from build123d import *

# Parameters (mm, degrees)
F3_D           = 4.4
F3_CSINK_D     = 8.96
F3_CSINK_ANGLE = 90
F4_SIZE        = 1


with BuildPart() as f1:
    # F0 (on Front) → F1 (revolve)
    with BuildSketch(Plane.XZ):
        Polygon((0, 8), (0, 0), (3.5, 0), (3.5, 5), (7.5, 5), (7.5, 8), align=None)
    revolve(axis=Axis((0, 0, 4), (0, 0, 1)))

    # F3 (through all)
    with Locations(Plane.XY.offset(8)):
        with Locations((0, 0)):
            CounterSinkHole(F3_D / 2, F3_CSINK_D / 2, counter_sink_angle=F3_CSINK_ANGLE)

    # F4
    f4_edges = [f1.edges().sort_by_distance(p)[0] for p in [
        (-7.5, 0, 5),
    ]]
    chamfer(f4_edges, length=F4_SIZE)


solid = f1.part
Input: part model. Units: mm. Frame: model coordinates. A direction names the side the tool comes from. Give positions to 0.01 mm unless a question says otherwise; leave off trailing zeros. Write each loop counter-clockwise with the first axis right and the second up, starting at its lowest first coordinate (ties: lowest second). Pieces come first, ordered by that corner, then holes.
Q1. Section A-A, the plane x = 0. Output: boundary loops of the cut face in (y, z).
Q2. Material intervals for probe 1 along Y at (x, z) = (0, 3.15); probe 2 along Z at (x, y) = (5, 2); probe 3 along Y at (x, z) = (-0.75, 6.25), sorted ascending.
Q3. First-contact query: P1, Ø3, axis at x = 1, z = 1.5, coming from the +Y side; P2, Ø2.5, axis at x = 0, y = 0, coming from the -Z side; P3, Ø1, axis at y = -5.5, z = 5, coming from the +X side; P4, Ø3, axis at x = 4, y = 6, coming from the -Z side. Flat tips, straight axial feed; report the tip coordinate or a pass-through.
Q4. Pull-direction query (Y, two-part tool) for faces 1 (the face through (-3, -3, 5)), 2 (the face through (-2.1, 0.66, 2.82)), 3 (the face through (-7.493, 0.33, 7.014)); classes: pulls with the +Y half, pulls with the -Y half, needs draft (parallel to the pull), parting line crosses it, or undercut.
Q5. Section D-D, the plane z = 4.5. Output: boundary loops of the cut face in (x, y).
Q6. Set-up query: faces 4 (the face through (3.233, -1.341, 2.535)), 5 (the face through (2, -2, 0)). Return all of +Z, -Z, +X, -X, +Y, -Y with unobstructed straight access to the full face (end or side cutting, diameter ignored); none if empty.
Q7. Section C-C, the plane z = 7. Output: boundary loops of the cut face in (x, y), plus the area to 3 significant figures.
Filled in:
1. outline: (-7.5, 6) - (-6.5, 5) - (-3.5, 5) - (-3.5, 0) - (-2.2, 0) - (-2.2, 5.72) - (-4.48, 8) - (-7.5, 8) - close; (2.2, 0) - (3.5, 0) - (3.5, 5) - (6.5, 5) - (7.5, 6) - (7.5, 8) - (4.48, 8) - (2.2, 5.72) - close
2. probe 1: y = -3.5 to -2.2, 2.2 to 3.5
2. probe 2: z = 5 to 8
2. probe 3: y = -7.46 to -2.62, 2.62 to 7.46
3. P1: stops at y = 3.5
3. P2: passes through
3. P3: stops at x = 4.54
3. P4: stops at z = 5
4. face 1: needs draft
4. face 2: undercut
4. face 3: parting line crosses it
5. outline: circle Ø7 at (0, 0); hole circle Ø4.4 at (0, 0)
6. face 4: -Z
6. face 5: -Z, +X, -X, +Y, -Y
7. outline: circle Ø15 at (0, 0); hole circle Ø6.96 at (0, 0)
7. area: 139 mm2
